```python
from build123d import *

# Parameters (mm, degrees)
SKETCH1_W           = 131
SKETCH1_H           = 85.8357277
SKETCH1_R           = 1.6
SKETCH1_R_2         = 2.1
SKETCH1_R_3         = 1.75
SKETCH1_R_4         = 25.65
SKETCH1_W_2         = 21.5
SKETCH1_H_2         = 42
BOSS_EXTRUDE1_DEPTH = 5


with BuildPart() as part:
    # Sketch1 → Boss-Extrude1 (new body)
    with BuildSketch(Plane(origin=(0, 0, 0), x_dir=(1, 0, 0), z_dir=(0, 1, 0))):
        with Locations((0, -0.385889954)):
            Rectangle(SKETCH1_W, SKETCH1_H)
        with Locations(Location((-55.5, -26, 0), (0, 0, 270))):
            Circle(SKETCH1_R, mode=Mode.SUBTRACT)
        with Locations(Location((-60, -40, 0), (0, 0, 270))):
            Circle(SKETCH1_R, mode=Mode.SUBTRACT)
        with Locations(Location((60, -40, 0), (0, 0, 270))):
            Circle(SKETCH1_R, mode=Mode.SUBTRACT)
        with Locations(Location((60, 40, 0), (0, 0, 270))):
            Circle(SKETCH1_R, mode=Mode.SUBTRACT)
        with Locations(Location((45, 34.25, 0), (0, 0, 270))):
            Circle(SKETCH1_R_2, mode=Mode.SUBTRACT)
        with Locations(Location((55, 34.25, 0), (0, 0, 270))):
            Circle(SKETCH1_R_2, mode=Mode.SUBTRACT)
        with Locations(Location((-55.5, 26, 0), (0, 0, 270))):
            Circle(SKETCH1_R_3, mode=Mode.SUBTRACT)
        with Locations(Location((45, -14.25, 0), (0, 0, 270))):
            Circle(SKETCH1_R_2, mode=Mode.SUBTRACT)
        with Locations(Location((-10, 0, 0), (0, 0, 270))):
            Circle(SKETCH1_R_4, mode=Mode.SUBTRACT)
        with Locations(Location((-60, 40, 0), (0, 0, 270))):
            Circle(SKETCH1_R, mode=Mode.SUBTRACT)
        with Locations(Location((55, -14.25, 0), (0, 0, 270))):
            Circle(SKETCH1_R_2, mode=Mode.SUBTRACT)
        with Locations((50, 10)):
            Rectangle(SKETCH1_W_2, SKETCH1_H_2, mode=Mode.SUBTRACT)
    extrude(amount=BOSS_EXTRUDE1_DEPTH)


solid = part.part
```
The listing builds one solid part. Answer for the finished solid, in the listing's coordinates (mm). A direction names the side the tool comes from. Coordinates: 2 decimals unless noted, no trailing zeros. Loops run counter-clockwise (first coordinate to the right, second up) from the corner with the lowest first, then second, coordinate; pieces in that order, holes last. Notation, with made-up numbers: (-25.75, -36.5) -> (-20.75, -36.5) arc R21 ccw to (-20.75, -32.5) -> close; hole circle Ø10 at (-4.75, -22). An arc over 180 degrees is marked (long way). Return JSON: item names as keys, results as strings. Group by question number.
(1) A cutting plane is placed at C-C on y = 3.8. Count the separate pieces of the cut face and the enclosed holes in it, and give its area (3 significant figures).
(2) A cutting plane is placed at B-B on x = 45. Write down the section's boundary in (y, z).
(3) Find the intervals of material crossed by probe 1 along X at (y, z) = (1.6, -34.25); probe 2 along X at (y, z) = (2.4, -33); probe 3 along Z at (x, y) = (46, 1.8), in increasing order. Write a range as from..to.
(4) Determine the mould class of faces 1 (the flat face through (-1, 2, 43.304)), 2 (the cylindrical face through (-56.56, 2.46, -27.39)), 3 (the flat face through (-1, 2, -42.532)), 4 (the cylindrical face through (-32.756, 2.465, 11.836)) for opening direction Z: released by +Z, released by -Z, zero draft, split by the parting line, or undercut.
(5) Which of the six approach directions +Z, -Z, +X, -X, +Y, -Y give full straight-line access (tool end or side, diameter ignored) to faces 5 (the flat face through (-65.5, 2, 1)), 6 (the flat face through (50, 2, 11))?
(6) A cutting plane is placed at D-D on x = -60. Write down the section's boundary in (y, z).
(7) A cutting plane is placed at A-A on z = -40. Write down the section's boundary in (x, y), and give its area (3 significant figures).
The answers:
{
 "1": {"separate pieces": "1", "enclosed holes": "12", "area": "8,170 mm^2"},
 "2": {"outline": "(0, -42.53) -> (5, -42.53) -> (5, -36.35) -> (0, -36.35) -> close; (0, -32.15) -> (5, -32.15) -> (5, -31) -> (0, -31) -> close; (0, 11) -> (5, 11) -> (5, 12.15) -> (0, 12.15) -> close; (0, 16.35) -> (5, 16.35) -> (5, 43.3) -> (0, 43.3) -> close"},
 "3": {"probe 1": "x = -65.5..42.9, 47.1..52.9, 57.1..65.5", "probe 2": "x = -65.5..43.31, 46.69..53.31, 56.69..65.5", "probe 3": "z = -42.53..-36.1, -32.4..-31, 11..12.4, 16.1..43.3"},
 "4": {"face 1": "released by +Z", "face 2": "undercut", "face 3": "released by -Z", "face 4": "undercut"},
 "5": {"face 5": "+Z, -Z, -X, +Y, -Y", "face 6": "+Y, -Y"},
 "6": {"outline": "(0, -42.53) -> (5, -42.53) -> (5, -41.6) -> (0, -41.6) -> close; (0, -38.4) -> (5, -38.4) -> (5, 38.4) -> (0, 38.4) -> close; (0, 41.6) -> (5, 41.6) -> (5, 43.3) -> (0, 43.3) -> close"},
 "7": {"outline": "(-65.5, 0) -> (-61.6, 0) -> (-61.6, 5) -> (-65.5, 5) -> close; (-58.4, 0) -> (58.4, 0) -> (58.4, 5) -> (-58.4, 5) -> close; (61.6, 0) -> (65.5, 0) -> (65.5, 5) -> (61.6, 5) -> close", "area": "623 mm^2"}
}
